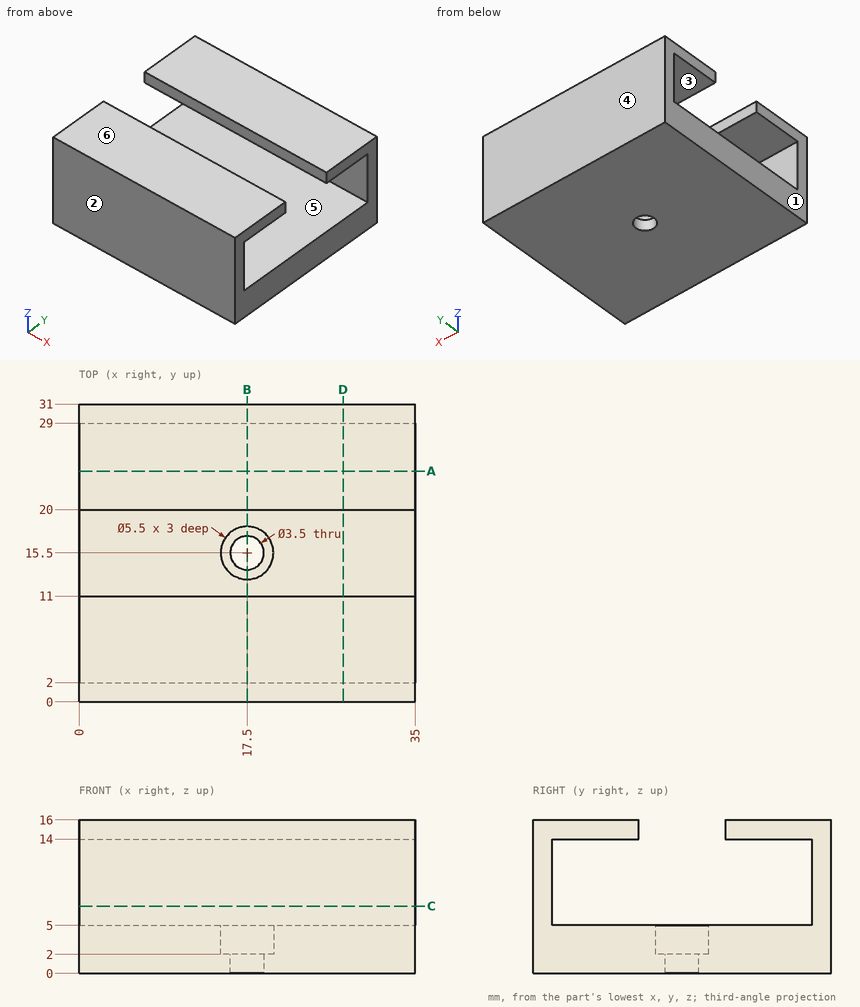
The figure shows three views and two pictorial views of one solid part (mm, origin at its lowest corner). Answer the questions. A direction names the side the tool comes from. Coordinates: 2 decimals unless noted, no trailing zeros. Write each loop counter-clockwise with the first axis right and the second up, starting at its lowest first coordinate (ties: lowest second). Pieces come first, ordered by that corner, then holes. Notation, with made-up numbers: (58.25, 80.25) -> (110.25, 80.25) arc R11 cw to (110.25, 95.25) -> close; hole circle Ø6 at (68.25, -13.5). An arc over 180 degrees is marked (long way). Return JSON: item names as keys, results as strings.
1. A cutting plane is placed at B-B (x = 17.5). Determine the outline of the cut face in (y, z).
Found:
{"outline": "(0, 0) -> (13.75, 0) -> (13.75, 2) -> (12.75, 2) -> (12.75, 5) -> (2, 5) -> (2, 14) -> (11, 14) -> (11, 16) -> (0, 16) -> close; (17.25, 0) -> (31, 0) -> (31, 16) -> (20, 16) -> (20, 14) -> (29, 14) -> (29, 5) -> (18.25, 5) -> (18.25, 2) -> (17.25, 2) -> close"}
2. Each of these flat-tipped pins is pushed along its axis until it touches: P1, Ø6.5, axis at x = 17.5, y = 15.5, coming from the -Z side; P2, Ø4, axis at x = 17.5, y = 15.5, coming from the +Z side; P3, Ø1.6, axis at x = 18, y = 16, coming from the +Z side. Where does it stop, or does it pass through?
Found:
{"P1": "z = 0", "P2": "z = 2", "P3": "through"}
3. A cutting plane is placed at C-C (z = 7). Determine the outline of the cut face in (x, y), and give its area (3 significant figures).
Found:
{"outline": "(0, 0) -> (35, 0) -> (35, 2) -> (0, 2) -> close; (0, 29) -> (35, 29) -> (35, 31) -> (0, 31) -> close", "area": "140 mm2"}
4. A cutting plane is placed at D-D (x = 27.5). Determine the outline of the cut face in (y, z), and give its area (3 significant figures).
Found:
{"outline": "(0, 0) -> (31, 0) -> (31, 16) -> (20, 16) -> (20, 14) -> (29, 14) -> (29, 5) -> (2, 5) -> (2, 14) -> (11, 14) -> (11, 16) -> (0, 16) -> close", "area": "235 mm2"}
5. Determine the mould class of the marked faces 1, 2, 3 and 4 for opening direction Y: pulls with the +Y half, pulls with the -Y half, needs draft (parallel to the pull), parting line crosses it, or undercut.
Found:
{"face 1": "needs draft", "face 2": "pulls with the -Y half", "face 3": "undercut", "face 4": "pulls with the +Y half"}
6. Find the intervals of material crossed by line 1 along Y through (x, z) = (13, 6); line 2 along Y through (x, z) = (17.5, 0.75); line 3 along Z through (x, y) = (4, 23), in increasing order. Write a range as from..to.
Found:
{"line 1": "0..2, 29..31", "line 2": "0..13.75, 17.25..31", "line 3": "0..5, 14..16"}
7. A cutting plane is placed at A-A (y = 24). Determine the outline of the cut face in (x, z).
Found:
{"outline": "(0, 0) -> (35, 0) -> (35, 5) -> (0, 5) -> close; (0, 14) -> (35, 14) -> (35, 16) -> (0, 16) -> close"}
8. A tool of negligible diameter and unlimited length cuts with its end or side. For the marked faces 5 and 6, from which of +Z, -Z, +X, -X, +Y, -Y can it reach the whole face along a straight path? Write none if from no direction.
Found:
{"face 5": "+X, -X", "face 6": "+Z, +X, -X, +Y, -Y"}
